Check sheet for the modelled part. Datum: model origin and axes. Units: mm. Coordinates: 2 decimals unless noted, no trailing zeros. Loops run counter-clockwise (first coordinate to the right, second up) from the corner with the lowest first, then second, coordinate; pieces in that order, holes last. Notation, with made-up numbers: (-3, -23.5) -> (18, -23.5) arc R35 ccw to (18, 8.5) -> close; hole circle Ø11 at (14, 14). An arc over 180 degrees is marked (long way). Use one line per item in the form item = value.
from build123d import *

# Parameters (mm, degrees)
CROQUIS3_W              = 150
CROQUIS3_H              = 50
SALIENTE_EXTRUIR3_DEPTH = 10
CROQUIS4_R              = 5
SALIENTE_EXTRUIR4_DEPTH = 8


with BuildPart() as part:
    # Croquis3 → Saliente-Extruir3 (new body)
    with BuildSketch(Plane.XY):
        Rectangle(CROQUIS3_W, CROQUIS3_H)
        with BuildLine():
            Line((60, 5), (-10, 5))
            ThreePointArc((-10, 5), (-15, 0), (-10, -5))
            Line((-10, -5), (60, -5))
            ThreePointArc((60, -5), (65, 0), (60, 5))
        make_face(mode=Mode.SUBTRACT)
    extrude(amount=SALIENTE_EXTRUIR3_DEPTH)

    # Croquis4 → Saliente-Extruir4 (add)
    with BuildSketch(Plane.XY.offset(10)):
        with Locations((-50, 0)):
            Circle(CROQUIS4_R)
    extrude(amount=SALIENTE_EXTRUIR4_DEPTH)


solid = part.part
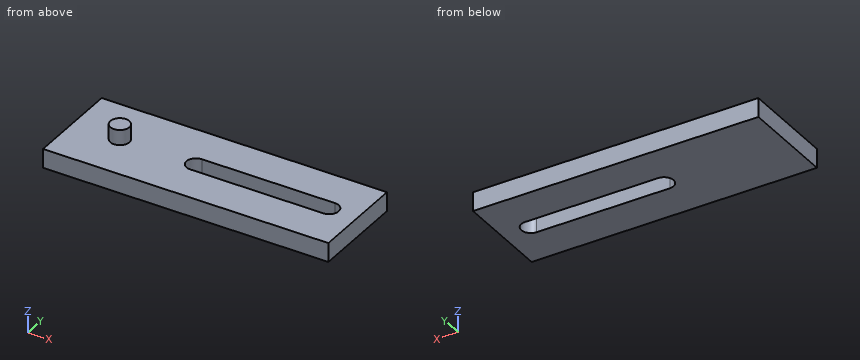
(1) Section check A-A, the plane z = 5.75. Record the boundary of the cut face in (x, y).
Established:
outline = (-75, -25) -> (75, -25) -> (75, 25) -> (-75, 25) -> close; hole (-10, -5) -> (60, -5) arc R5 ccw to (60, 5) -> (-10, 5) arc R5 ccw to start
(2) Go/stop test with a flat-tipped pin: P1, Ø5, axis at x = 26.5, z = 13.5, coming from the -Y side. Record where the tip stops, or that it passes through.
Established:
P1 = through
(3) Section check C-C, the plane x = 53.5. Record the boundary of the cut face in (y, z), plus the area to 3 significant figures.
Established:
outline = (-25, 0) -> (-5, 0) -> (-5, 10) -> (-25, 10) -> close; (5, 0) -> (25, 0) -> (25, 10) -> (5, 10) -> close
area = 400 mm²
(4) Section check B-B, the plane y = 0. Record the boundary of the cut face in (x, z), plus the area to 3 significant figures.
Established:
outline = (-75, 0) -> (-15, 0) -> (-15, 10) -> (-45, 10) -> (-45, 18) -> (-55, 18) -> (-55, 10) -> (-75, 10) -> close; (65, 0) -> (75, 0) -> (75, 10) -> (65, 10) -> close
area = 780 mm²
(5) Section check D-D, the plane x = -50. Record the boundary of the cut face in (y, z).
Established:
outline = (-25, 0) -> (25, 0) -> (25, 10) -> (5, 10) -> (5, 18) -> (-5, 18) -> (-5, 10) -> (-25, 10) -> close
(6) Scan lines: line 1 along Y through (x, z) = (33, 1.5); line 2 along X through (y, z) = (-4, 1); line 3 along Z through (x, y) = (-45, 2). Record each from-to range of solid material in increasing order.
Established:
line_1 = -25 to -5, 5 to 25
line_2 = -75 to -13, 63 to 75
line_3 = 0 to 10
